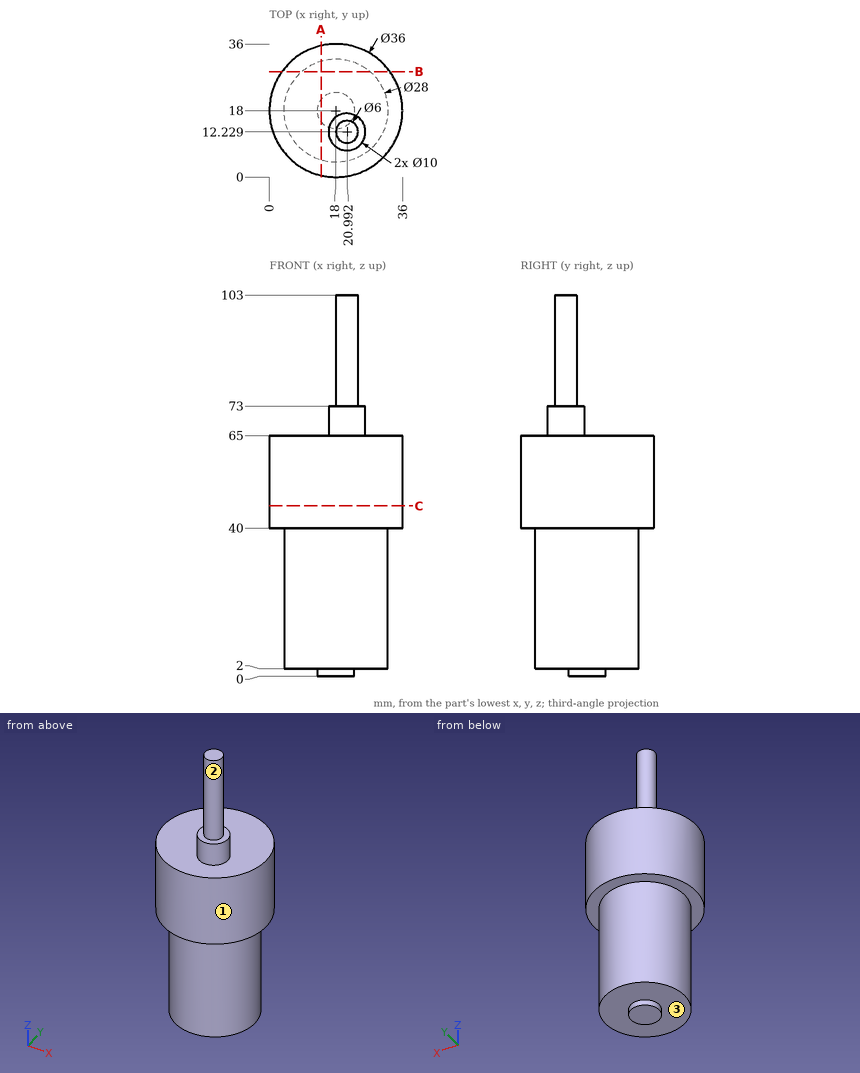
Geometry: see drawing. Coordinates: mm, zero at the bounding-box minimum. A direction names the side the tool comes from. Coordinates: 2 decimals unless noted, no trailing zeros. Loops run counter-clockwise (first coordinate to the right, second up) from the corner with the lowest first, then second, coordinate; pieces in that order, holes last. Notation, with made-up numbers: (42, 22) - (84, 22) arc R32 ccw to (84, 48) - close; hole circle Ø10 at (84, 79.5). An arc over 180 degrees is marked (long way). Answer in a Markdown table with one row per item.
(1) Cut plane A-A on x = 14. Output: boundary loops of the cut face in (y, z).
Model answer:
| item | result |
|---|---|
| outline | (0.45, 40) - (4.58, 40) - (4.58, 2) - (15, 2) - (15, 0) - (21, 0) - (21, 2) - (31.42, 2) - (31.42, 40) - (35.55, 40) - (35.55, 65) - (0.45, 65) - close |
(2) Cut plane B-B on y = 28.5. Output: boundary loops of the cut face in (x, z).
Model answer:
| item | result |
|---|---|
| outline | (3.38, 40) - (8.74, 40) - (8.74, 2) - (27.26, 2) - (27.26, 40) - (32.62, 40) - (32.62, 65) - (3.38, 65) - close |
(3) Cut plane C-C on z = 46. Output: boundary loops of the cut face in (x, y).
Model answer:
| item | result |
|---|---|
| outline | circle Ø36 at (18, 18) |
(4) Pin query (flat end, axial travel): P1, Ø10, axis at x = 16.5, z = 35.5, coming from the -Y side; P2, Ø5, axis at y = 26.5, z = 44, coming from the -X side; P3, Ø1, axis at x = 24.5, z = 29, coming from the +Y side. Return the tip coordinate at first contact, or that it passes through.
Model answer:
| item | result |
|---|---|
| P1 | stops at y = 0 |
| P2 | stops at x = 1.03 |
| P3 | stops at y = 30.65 |
(5) Material intervals for L1, parallel to Y at x = 17.5, z = 39; L2, parallel to Z at x = 10, y = 5; L3, parallel to Z at x = 8, y = 27.5, sorted ascending. Write a range as from..to.
Model answer:
| item | result |
|---|---|
| L1 | y = 4.01..31.99 |
| L2 | z = 40..65 |
| L3 | z = 2..65 |
(6) Set-up query: the marked faces 1, 2 and 3. Return all of +Z, -Z, +X, -X, +Y, -Y with unobstructed straight access to the full face (end or side cutting, diameter ignored); none if empty.
Model answer:
| item | result |
|---|---|
| face 1 | +Z, -Z |
| face 2 | +Z |
| face 3 | -Z |
